Geometry: see drawing. Coordinates: mm, zero at the bounding-box minimum. A direction names the side the tool comes from. Coordinates: 2 decimals unless noted, no trailing zeros. Write each loop counter-clockwise with the first axis right and the second up, starting at its lowest first coordinate (ties: lowest second). Pieces come first, ordered by that corner, then holes. Notation, with made-up numbers: (-26.5, -5) -> (-12.5, -5) arc R12 cw to (-12.5, 9) -> close; hole circle Ø8 at (-19, 54). An arc over 180 degrees is marked (long way). Answer as a JSON object with one key per item and string values. Group by question number.
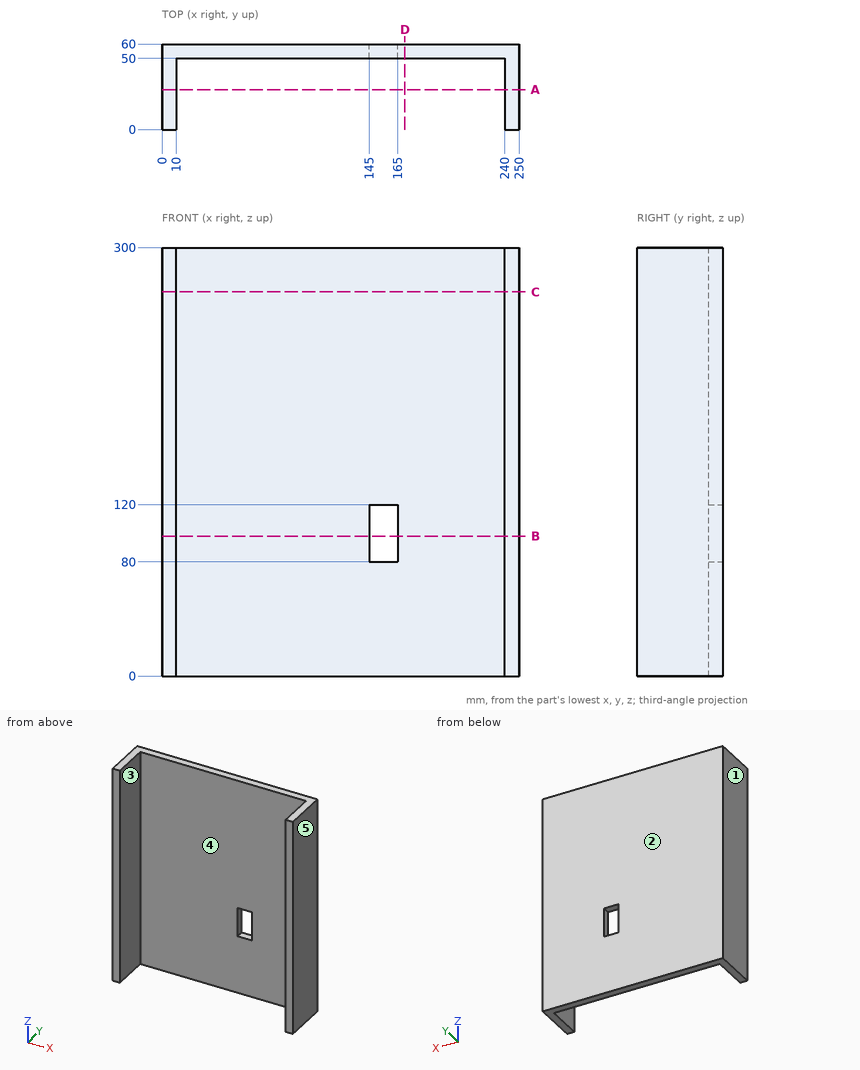
Item 1: Set-up query: the marked faces 4 and 5. Return all of +Z, -Z, +X, -X, +Y, -Y with unobstructed straight access to the full face (end or side cutting, diameter ignored); none if empty.
Item 2: Mould query, pull axis X, two halves, no side actions, for the marked faces 1, 2 and 3. Classes: +X half, -X half, draft (parallel to the pull), parting line (faces both ways), or undercut.
Item 3: Section A-A on y = 28. Output: boundary loops of the cut face in (x, z), then the cut area to 3 significant figures.
Item 4: Section D-D on x = 170. Output: boundary loops of the cut face in (y, z), then the cut area to 3 significant figures.
Item 5: Section B-B on z = 98. Output: boundary loops of the cut face in (x, y).
Item 6: Section C-C on z = 269. Output: boundary loops of the cut face in (x, y), then the cut area to 3 significant figures.
Item 7: Contact query for a flat-ended pin moving along its axis: pin 1 (10 mm diameter, centred on x = 41, z = 161.5, fed in from -Y). Output: stop coordinate, or through.
Item 8: Ray query, L1, parallel to Z at x = 149, y = 51; L2, parallel to X at y = 27, z = 116; L3, parallel to Y at x = 137, z = 244. Return the intervals inside material, ascending. Write a range as [from, to].
Answer sheet:
{
 "1": {"face 4": "+Z, -Z, -Y", "face 5": "+Z, -Z, +X, +Y, -Y"},
 "2": {"face 1": "-X half", "face 2": "draft", "face 3": "undercut"},
 "3": {"outline": "(0, 0) -> (10, 0) -> (10, 300) -> (0, 300) -> close; (240, 0) -> (250, 0) -> (250, 300) -> (240, 300) -> close", "area": "6,000 mm^2"},
 "4": {"outline": "(50, 0) -> (60, 0) -> (60, 300) -> (50, 300) -> close", "area": "3,000 mm^2"},
 "5": {"outline": "(0, 0) -> (10, 0) -> (10, 50) -> (145, 50) -> (145, 60) -> (0, 60) -> close; (165, 50) -> (240, 50) -> (240, 0) -> (250, 0) -> (250, 60) -> (165, 60) -> close"},
 "6": {"outline": "(0, 0) -> (10, 0) -> (10, 50) -> (240, 50) -> (240, 0) -> (250, 0) -> (250, 60) -> (0, 60) -> close", "area": "3,500 mm^2"},
 "7": {"pin 1": "stops at y = 50"},
 "8": {"L1": "z = [0, 80], [120, 300]", "L2": "x = [0, 10], [240, 250]", "L3": "y = [50, 60]"}
}
